The listing builds one solid part. Answer for the finished solid, in the listing's coordinates (mm). A direction names the side the tool comes from. Coordinates: 2 decimals unless noted, no trailing zeros. Write each loop counter-clockwise with the first axis right and the second up, starting at its lowest first coordinate (ties: lowest second). Pieces come first, ordered by that corner, then holes.
(1) The part is cut by section A-A on y = 18.5. Determine the outline of the cut face in (x, z), plus the area to 3 significant figures.
(2) Given P1, Ø1.6, axis at x = 0, z = -13, coming from the -Y side; P2, Ø1, axis at x = 6, z = -8, coming from the -Y side; P3, Ø6, axis at x = 6, y = 17, coming from the +Z side; P4, Ø10.5, axis at x = -4, z = 7.5, coming from the +Y side, each flat-ended and moving along its own axis, determine where each tip first touches the part or whether it passes through.
(3) The part is cut by section C-C on y = 8.5. Determine the outline of the cut face in (x, z).
(4) Straight lines are drawn through the part: line 1 (X direction, y = 15.55, z = -6.35); line 2 (X direction, y = 11.75, z = -7.5); line 3 (X direction, y = 25.6, z = 0). For each, find the intervals that lie inside material, in ascending order.
(5) The part is cut by section B-B on y = 24.5. Determine the outline of the cut face in (x, z), plus the area to 3 significant figures.
(6) Which of the six approach directions +Z, -Z, +X, -X, +Y, -Y give full straight-line access (tool end or side, diameter ignored) to faces 1 (the conical face through (3.8, 9.36, -1.2)), 2 (the cylindrical face through (-7.141, 23.023, -22.677))?
(7) For a pull along Z with two mould halves and no side action, classify faces 3 (the cylindrical face through (22.4, 17.9, -11.7)), 4 (the conical face through (10.922, 16.034, 6.34)) as +Z half, -Z half, draft (parallel to the pull), parting line (faces both ways), or undercut.
from build123d import *

# Parameters (mm, degrees)
CHAMFER1_SIZE      = 0.381
CHAMFER2_SIZE      = 0.762
CHAMFER4_SIZE      = 1.27
SKETCH3_R          = 1.5875
SKETCH2_R          = 4.7625
SKETCH5_R          = 2.4384
SKETCH4_R          = 6.35
SKETCH9_R          = 2.4384
CUT_EXTRUDE1_DEPTH = 1.27
SKETCH3_3_R        = 1.5875
CUT_EXTRUDE2_DEPTH = 0.381
SKETCH14_R         = 2.4384
SKETCH12_R         = 6.35
SKETCH16_R         = 1.5875
SKETCH15_R         = 4.7625
CIRPATTERN2_COUNT  = 6
SKETCH17_R         = 1.5875
CUT_EXTRUDE4_DEPTH = 25.4


with BuildPart() as part:
    # Sketch1 → Revolve1 (revolve)
    with BuildSketch(Plane.XY, mode=Mode.PRIVATE) as revolve1_sk:
        Polygon((0, 20.6756), (0, 0), (19.05, 0), (19.05, 14.5288), (22.2123, 14.5288), (22.2123, 16.3068), (25.273, 16.3068), (25.273, 19.4818), (23.7744, 19.4818), (23.7744, 26.4668), (21.1074, 26.4668), (21.1074, 23.8252), (17.4625, 20.6756), align=None)
    revolve(revolve1_sk.sketch.rotate(Axis((0, 0, 0), (0, 1, 0)), 90), axis=Axis((0, 0, 0), (0, 1, 0)))

    # Chamfer1
    chamfer1_edges = [part.edges().sort_by_distance(p)[0] for p in [
        (0, 26.4668, 21.1074),
    ]]
    chamfer(chamfer1_edges, length=CHAMFER1_SIZE)

    # Chamfer2
    chamfer2_edges = [part.edges().sort_by_distance(p)[0] for p in [
        (0, 0, 19.05),
    ]]
    chamfer(chamfer2_edges, length=CHAMFER2_SIZE)

    # Chamfer4
    chamfer4_edges = [part.edges().sort_by_distance(p)[0] for p in [
        (0, 14.5288, 19.05),
    ]]
    chamfer(chamfer4_edges, length=CHAMFER4_SIZE)

    # Sketch3 → Cut-Loft1 section 0
    with BuildSketch(Plane(origin=(0, 16.764, 0), x_dir=(1, 0, 0), z_dir=(0, 1, 0))):
        with Locations((0, 12.7)):
            Circle(SKETCH3_R)
    # Sketch2 → Cut-Loft1 section 1
    with BuildSketch(Plane(origin=(0, 20.6756, 0), x_dir=(1, 0, 0), z_dir=(0, 1, 0))):
        with Locations((0, 12.7)):
            Circle(SKETCH2_R)
    cut_loft1 = loft(mode=Mode.SUBTRACT)

    # Sketch5 → Cut-Loft3 section 0
    with BuildSketch(Plane(origin=(0, 16.764, 0), x_dir=(1, 0, 0), z_dir=(0, 1, 0))):
        Circle(SKETCH5_R)
    # Sketch4 → Cut-Loft3 section 1
    with BuildSketch(Plane(origin=(0, 20.6756, 0), x_dir=(1, 0, 0), z_dir=(0, 1, 0))):
        Circle(SKETCH4_R)
    loft(mode=Mode.SUBTRACT)

    # Sketch9 → Cut-Extrude1 (cut)
    with BuildSketch(Plane(origin=(0, 16.764, 0), x_dir=(1, 0, 0), z_dir=(0, 1, 0))):
        with Locations(Location((0, 0, 0), (0, 0, 270))):
            Circle(SKETCH9_R)
    extrude(amount=-CUT_EXTRUDE1_DEPTH, mode=Mode.SUBTRACT)

    # Sketch3_3 → Cut-Extrude2 (cut)
    with BuildSketch(Plane(origin=(0, 16.764, 0), x_dir=(1, 0, 0), z_dir=(0, 1, 0))):
        with Locations(Location((0, 12.7, 0), (0, 0, 270))):
            Circle(SKETCH3_3_R)
    cut_extrude2 = extrude(amount=-CUT_EXTRUDE2_DEPTH, mode=Mode.SUBTRACT)

    # Cut-Extrude3 cone 1 section (through the dimple's axis) → Cut-Extrude3 (revolve, cut)
    with BuildSketch(Plane(origin=(0, 16.383, -12.7), x_dir=(0, 0, 1), z_dir=(1, 0, 0))):
        Polygon((0, 0), (1.5875, 0), (0, 0.366503253), align=None)
    cut_extrude3 = revolve(axis=Axis((0, 16.383, -12.7), (0, -1, 0)), mode=Mode.SUBTRACT)

    # Sketch14 → Cut-Loft5 section 0
    with BuildSketch(Plane(origin=(0, 15.494, 0), x_dir=(1, 0, 0), z_dir=(0, 1, 0))):
        Circle(SKETCH14_R)
    # Sketch12 → Cut-Loft5 section 1
    with BuildSketch(Plane.XZ):
        Circle(SKETCH12_R)
    loft(mode=Mode.SUBTRACT)

    # Sketch16 → Cut-Loft7 section 0
    with BuildSketch(Plane(origin=(0, 12.573, 0), x_dir=(-1, 0, 0), z_dir=(0, -1, 0))):
        with Locations((0, 12.7)):
            Circle(SKETCH16_R)
    # Sketch15 → Cut-Loft7 section 1
    with BuildSketch(Plane.XZ):
        with Locations((0, -12.7)):
            Circle(SKETCH15_R)
    cut_loft7 = loft(mode=Mode.SUBTRACT)

    # CirPattern2: Cut-Loft1, Cut-Extrude2, Cut-Extrude3, Cut-Loft7 ×6 about axis
    cirpattern2_axis = Axis((0, 0, 0), (0, 1, 0))
    add([cut_loft1.rotate(cirpattern2_axis, i * 360 / CIRPATTERN2_COUNT) for i in range(1, CIRPATTERN2_COUNT)], mode=Mode.SUBTRACT)
    add([cut_extrude2.rotate(cirpattern2_axis, i * 360 / CIRPATTERN2_COUNT) for i in range(1, CIRPATTERN2_COUNT)], mode=Mode.SUBTRACT)
    add([cut_extrude3.rotate(cirpattern2_axis, i * 360 / CIRPATTERN2_COUNT) for i in range(1, CIRPATTERN2_COUNT)], mode=Mode.SUBTRACT)
    add([cut_loft7.rotate(cirpattern2_axis, i * 360 / CIRPATTERN2_COUNT) for i in range(1, CIRPATTERN2_COUNT)], mode=Mode.SUBTRACT)

    # Sketch17 → Cut-Extrude4 (cut)
    with BuildSketch(Plane(origin=(0, 20.6756, 0), x_dir=(1, 0, 0), z_dir=(0, 1, 0))):
        with Locations(Location((-10.998522628, 6.35, 0), (0, 0, 330))):
            Circle(SKETCH17_R)
        with Locations(Location((10.998522628, 6.35, 0), (0, 0, 210))):
            Circle(SKETCH17_R)
        with Locations(Location((0, -12.7, 0), (0, 0, 270))):
            Circle(SKETCH17_R)
    extrude(amount=-CUT_EXTRUDE4_DEPTH, mode=Mode.SUBTRACT)


solid = part.part
Model answer:
1. outline: circle Ø50.55 at (0, 0); hole circle Ø5.99 at (-11, -6.35); hole circle Ø5.99 at (-11, 6.35); hole circle Ø8.35 at (0, 0); hole circle Ø5.99 at (0, -12.7); hole circle Ø5.99 at (0, 12.7); hole circle Ø5.99 at (11, -6.35); hole circle Ø5.99 at (11, 6.35)
1. area: 1,780 mm2
2. P1: stops at y = 12.57
2. P2: stops at y = 0
2. P3: stops at z = 25.09
2. P4: stops at y = 20.68
3. outline: circle Ø38.1 at (0, 0); hole circle Ø5.23 at (-11, -6.35); hole circle Ø5.23 at (-11, 6.35); hole circle Ø8.41 at (0, 0); hole circle Ø5.23 at (0, -12.7); hole circle Ø5.23 at (0, 12.7); hole circle Ø5.23 at (11, -6.35); hole circle Ø5.23 at (11, 6.35)
4. line 1: x = -21.29 to -12.59, -9.41 to 9.41, 12.59 to 21.29
4. line 2: x = -17.51 to -12.38, -9.62 to 9.62, 12.38 to 17.51
4. line 3: x = -23.77 to -21.11, 21.11 to 23.77
5. outline: circle Ø47.55 at (0, 0); hole circle Ø42.21 at (0, 0)
5. area: 376 mm2
6. face 1: -Y
6. face 2: +Y
7. face 3: parting line
7. face 4: undercut
